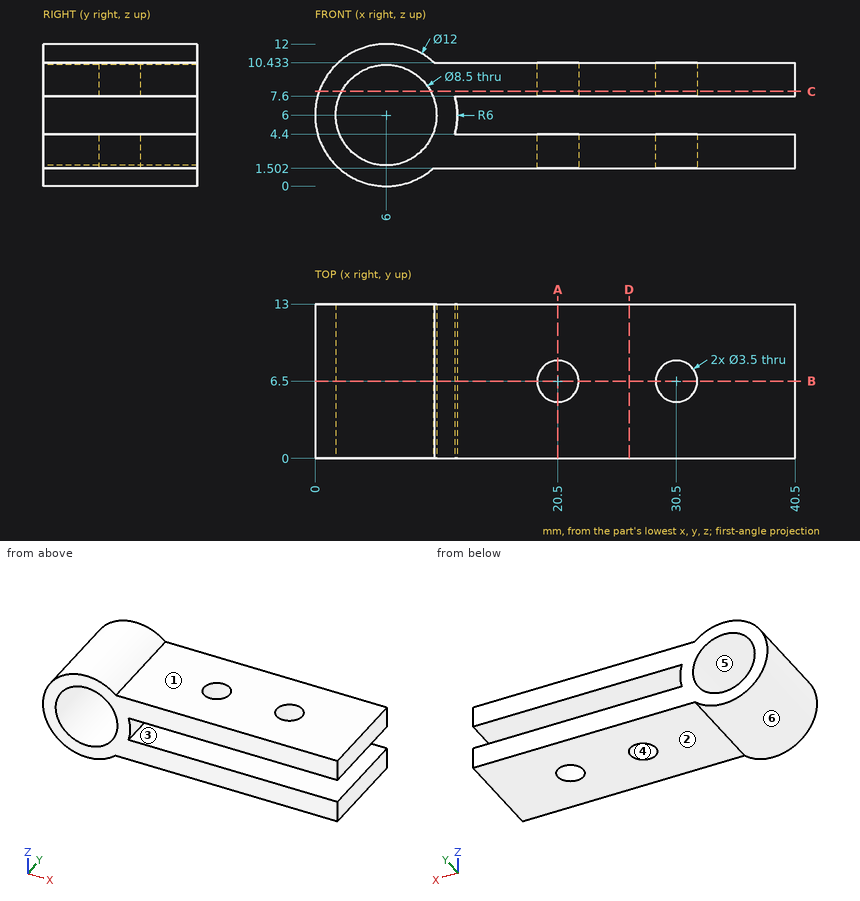
Geometry check sheet. Reference: drawing and pictorial views, mm from the part's lowest x, y, z. A direction names the side the tool comes from. Give positions to 0.01 mm unless a question says otherwise; leave off trailing zeros. Loops run counter-clockwise (first coordinate to the right, second up) from the corner with the lowest first, then second, coordinate; pieces in that order, holes last.
1. Section check B-B, the plane y = 6.5. Enter the section's corners in (x, z), then the cut area to 3 significant figures.
2. Go/stop test with flat-tipped pins: pin 1 Ø4 at (x, y) = (30.5, 6.5) entering from -Z; pin 2 Ø6.5 at (x, y) = (23, 5.5) entering from +Z. Record where each tip stops, or that it passes through.
3. Thickness scan on line 1 (Z direction, x = 12.5, y = 9.25); line 2 (Y direction, x = 30.5, z = 3.3); line 3 (X direction, y = 3.25, z = 5.75) (1 decimal). Record the ranges inside material, lowest first.
4. Set-up check for the marked faces 1, 2 and 3: record each of +Z, -Z, +X, -X, +Y, -Y from which the full face is reachable in a straight line by a thin tool's end or side.
5. Mould release check, pull along Z, two halves, no side actions. Record for the marked faces 4, 5 and 6: released by +Z, released by -Z, zero draft, split by the parting line, or undercut.
6. Section check C-C, the plane z = 8. Enter the section's corners in (x, y), then the cut area to 3 significant figures.
7. Section check A-A, the plane x = 20.5. Enter the section's corners in (y, z).
8. Section check D-D, the plane x = 26.5. Enter the section's corners in (y, z), then the cut area to 3 significant figures.
Geometry says:
1. outline: (9.97, 1.5) - (18.75, 1.5) - (18.75, 4.4) - (11.78, 4.4) arc R6 ccw to (11.78, 7.6) - (18.75, 7.6) - (18.75, 10.43) - (10.04, 10.43) arc R6 ccw (long way) to start; (22.25, 1.5) - (28.75, 1.5) - (28.75, 4.4) - (22.25, 4.4) - close; (22.25, 7.6) - (28.75, 7.6) - (28.75, 10.43) - (22.25, 10.43) - close; (32.25, 1.5) - (40.5, 1.5) - (40.5, 4.4) - (32.25, 4.4) - close; (32.25, 7.6) - (40.5, 7.6) - (40.5, 10.43) - (32.25, 10.43) - close; hole circle Ø8.5 at (6, 6)
1. area: 185 mm2
2. pin 1: stops at z = 1.5
2. pin 2: stops at z = 10.43
3. line 1: z = 1.5 to 4.4, 7.6 to 10.43
3. line 2: y = 0 to 4.75, 8.25 to 13
3. line 3: x = 0 to 1.8, 10.2 to 12
4. face 1: +Z, +X, +Y, -Y
4. face 2: -Z, +X, +Y, -Y
4. face 3: +X, +Y, -Y
5. face 4: zero draft
5. face 5: undercut
5. face 6: split by the parting line
6. outline: (0.34, 0) - (2.25, 0) - (2.25, 13) - (0.34, 13) - close; (9.75, 0) - (40.5, 0) - (40.5, 13) - (9.75, 13) - close; hole circle Ø3.5 at (20.5, 6.5); hole circle Ø3.5 at (30.5, 6.5)
6. area: 405 mm2
7. outline: (0, 1.5) - (4.75, 1.5) - (4.75, 4.4) - (0, 4.4) - close; (0, 7.6) - (4.75, 7.6) - (4.75, 10.43) - (0, 10.43) - close; (8.25, 1.5) - (13, 1.5) - (13, 4.4) - (8.25, 4.4) - close; (8.25, 7.6) - (13, 7.6) - (13, 10.43) - (8.25, 10.43) - close
8. outline: (0, 1.5) - (13, 1.5) - (13, 4.4) - (0, 4.4) - close; (0, 7.6) - (13, 7.6) - (13, 10.43) - (0, 10.43) - close
8. area: 74.5 mm2
